The listing builds one solid part. Answer for the finished solid, in the listing's coordinates (mm). Face numbers are marked on the shaded views. A direction names the side the tool comes from. Round coordinates to 2 decimals unless told otherwise and drop trailing zeros. Write each loop counter-clockwise with the first axis right and the second up, starting at its lowest first coordinate (ties: lowest second). Pieces come first, ordered by that corner, then holes.
Item 1: Find the intervals of material crossed by probe 1 along X at (y, z) = (-1.6, 14); probe 2 along Y at (x, z) = (-30, -7.5); probe 3 along Z at (x, y) = (-9, -3), in increasing order.
Item 2: Each of these flat-tipped pins is pushed along its axis until it touches: pin 1 (2.5 mm diameter, centred on x = -51.5, y = -1.5, fed in from +Z); pin 2 (4 mm diameter, centred on x = -22.5, z = 0, fed in from +Y); pin 3 (4 mm diameter, centred on x = 0, z = 0, fed in from +Y); pin 4 (1.5 mm diameter, centred on x = 6, z = 37.5, fed in from -Y). Where does it stop, or does it pass through?
Item 3: Find section C-C on x = -51.75. Give the vertices of the cut face in (y, z).
Item 4: A tool of negligible diameter and unlimited length cuts with its end or side. For the marked faces 1 and 2, from which of +Z, -Z, +X, -X, +Y, -Y can it reach the whole face along a straight path? Write none if from no direction.
Item 5: Find section B-B on z = -14. Give the vertices of the cut face in (x, y), then the cut area to 3 significant figures.
Item 6: Find section D-D on x = 14. Give the vertices of the cut face in (y, z).
```python
from build123d import *

# Parameters (mm, degrees)
SKETCH1_R                               = 50
BOSS_EXTRUDE1_DEPTH                     = 4.5
BOSS_EXTRUDE2_DEPTH                     = 5
SKETCH4_R                               = 18
SKETCH4_R_2                             = 16
EXTRUDE_THIN1_DEPTH                     = 5
SKETCH7_R                               = 27
CUT_EXTRUDE1_DEPTH                      = 2
CBORE_FOR_M5_HEX_HEAD_BOLT2_D           = 5
CBORE_FOR_M5_HEX_HEAD_BOLT2_CBORE_D     = 13
CBORE_FOR_M5_HEX_HEAD_BOLT2_CBORE_DEPTH = 2
CUT_EXTRUDE2_DEPTH                      = 74.247866863
SKETCH11_R                              = 2.5
BOSS_EXTRUDE3_DEPTH                     = 4
SKETCH12_R                              = 1
CUT_EXTRUDE3_DEPTH                      = 74.764829018
EXTRUDE_THIN2_REACH                     = 75.765
SKETCH13_R                              = 2.5
SKETCH13_R_2                            = 1.5
CIRPATTERN1_COUNT                       = 4
SKETCH14_R                              = 1.25
CUT_EXTRUDE4_DEPTH                      = 74.247866863


with BuildPart() as part:
    # Sketch1 → Boss-Extrude1 (new body)
    with BuildSketch(Plane(origin=(0, 0, 0), x_dir=(1, 0, 0), z_dir=(0, 1, 0))):
        with Locations(Location((0, 0, 0), (0, 0, 270))):
            Circle(SKETCH1_R)
    extrude(amount=BOSS_EXTRUDE1_DEPTH)

    # Sketch3 → Boss-Extrude2 (add, symmetric)
    with BuildSketch(Plane.XY):
        with BuildLine():
            Line((0, 2.5), (-53, 2.5))
            Line((-53, 2.5), (-53, -2.25))
            ThreePointArc((-53, -2.25), (-51.75, -3.5), (-50.5, -2.25))
            Line((-50.5, -2.25), (-50.5, 0))
            Line((-50.5, 0), (0, 0))
            Line((0, 0), (0, 2.5))
        make_face()
    extrude(amount=BOSS_EXTRUDE2_DEPTH, both=True)

    # Sketch4 → Extrude-Thin1 (add)
    with BuildSketch(Plane.XZ):
        Circle(SKETCH4_R)
        Circle(SKETCH4_R_2, mode=Mode.SUBTRACT)
    extrude(amount=EXTRUDE_THIN1_DEPTH)

    # Sketch7 → Cut-Extrude1 (cut)
    with BuildSketch(Plane(origin=(0, 4.5, 0), x_dir=(1, 0, 0), z_dir=(0, 1, 0))):
        with Locations(Location((0, 0, 0), (0, 0, 270))):
            Circle(SKETCH7_R)
    extrude(amount=-CUT_EXTRUDE1_DEPTH, mode=Mode.SUBTRACT)

    # CBORE for M5 Hex Head Bolt2 (through all)
    with Locations(Plane(origin=(0, 2.5, 0), x_dir=(1, 0, 0), z_dir=(0, 1, 0))):
        with Locations((0, 0)):
            CounterBoreHole(CBORE_FOR_M5_HEX_HEAD_BOLT2_D / 2, CBORE_FOR_M5_HEX_HEAD_BOLT2_CBORE_D / 2, CBORE_FOR_M5_HEX_HEAD_BOLT2_CBORE_DEPTH)

    # Sketch10 → Cut-Extrude2 (cut, through all)
    with BuildSketch(Plane(origin=(0, 2.5, 0), x_dir=(1, 0, 0), z_dir=(0, 1, 0))):
        with BuildLine():
            Line((-21.405668752, 16.455921283), (-23.792893219, 19.550252532))
            ThreePointArc((-23.792893219, 19.550252532), (-28.035533906, 28.035533906), (-19.550252532, 23.792893219))
            Line((-19.550252532, 23.792893219), (-16.455921283, 21.405668752))
            ThreePointArc((-16.455921283, 21.405668752), (-19.091883092, 19.091883092), (-21.405668752, 16.455921283))
        make_face()
    cut_extrude2 = extrude(amount=CUT_EXTRUDE2_DEPTH, mode=Mode.SUBTRACT)

    # Sketch11 → Boss-Extrude3 (add)
    with BuildSketch(Plane(origin=(0, 2.5, 0), x_dir=(1, 0, 0), z_dir=(0, 1, 0))):
        with Locations(Location((-24.5, 24.5, 0), (0, 0, 270))):
            Circle(SKETCH11_R)
    boss_extrude3 = extrude(amount=BOSS_EXTRUDE3_DEPTH)

    # Sketch12 → Cut-Extrude3 (cut, through all)
    with BuildSketch(Plane(origin=(0, 6.5, 0), x_dir=(1, 0, 0), z_dir=(0, 1, 0))):
        with Locations(Location((-24.5, 24.5, 0), (0, 0, 270))):
            Circle(SKETCH12_R)
    cut_extrude3 = extrude(amount=-CUT_EXTRUDE3_DEPTH, mode=Mode.SUBTRACT)

    # Sketch13 → Extrude-Thin2 (add, up to next)
    with BuildSketch(Plane.XZ.offset(5), mode=Mode.PRIVATE) as extrude_thin2_sk1:
        with Locations((-14, 0)):
            Circle(SKETCH13_R)
        with Locations((-14, 0)):
            Circle(SKETCH13_R_2, mode=Mode.SUBTRACT)
    extrude_thin2_tool1 = extrude(extrude_thin2_sk1.sketch, amount=-EXTRUDE_THIN2_REACH, mode=Mode.PRIVATE) - part.part
    extrude_thin2 = extrude_thin2_tool1.solids().sort_by_distance((-16.429289, -5, 0))[0]
    add(extrude_thin2)

    # CirPattern1: Cut-Extrude2, Boss-Extrude3, Cut-Extrude3, Extrude-Thin2 ×4 about axis
    cirpattern1_axis = Axis((0, 0, 0), (0, 1, 0))
    add([cut_extrude2.rotate(cirpattern1_axis, i * 360 / CIRPATTERN1_COUNT) for i in range(1, CIRPATTERN1_COUNT)], mode=Mode.SUBTRACT)
    add([boss_extrude3.rotate(cirpattern1_axis, i * 360 / CIRPATTERN1_COUNT) for i in range(1, CIRPATTERN1_COUNT)])
    add([cut_extrude3.rotate(cirpattern1_axis, i * 360 / CIRPATTERN1_COUNT) for i in range(1, CIRPATTERN1_COUNT)], mode=Mode.SUBTRACT)
    add([extrude_thin2.rotate(cirpattern1_axis, i * 360 / CIRPATTERN1_COUNT) for i in range(1, CIRPATTERN1_COUNT)])

    # Sketch14 → Cut-Extrude4 (cut, through all)
    with BuildSketch(Plane(origin=(0, 2.5, 0), x_dir=(1, 0, 0), z_dir=(0, 1, 0))):
        with Locations(Location((-23, 0, 0), (0, 0, 270))):
            Circle(SKETCH14_R)
    extrude(amount=-CUT_EXTRUDE4_DEPTH, mode=Mode.SUBTRACT)


solid = part.part
```
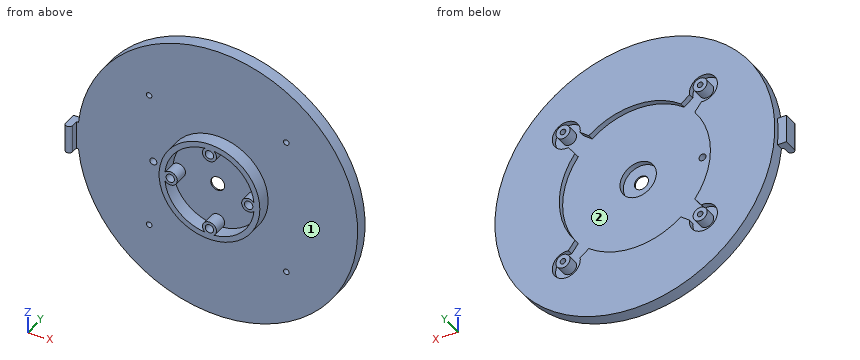
Check values:
1. probe 1: x = -11.31 to -7.75, -2.5 to -1.5, 1.5 to 2.5, 7.75 to 11.31
1. probe 2: y = 0 to 4.5
1. probe 3: z = -15.59 to -13.23, 13.23 to 15.59
2. pin 1: stops at z = 5
2. pin 2: stops at y = 2.5
2. pin 3: passes through
2. pin 4: stops at y = 0
3. outline: (-3.5, -5) - (2.5, -5) - (2.5, 5) - (-3.5, 5) - close
4. face 1: -Y
4. face 2: +Y
5. outline: (-48, 0) - (-11.31, 0) - (-11.31, -5) - (-7.75, -5) - (-7.75, 0) - (-2.5, 0) - (-2.5, -5) - (-1.5, -5) - (-1.5, 0) - (1.5, 0) - (1.5, -5) - (2.5, -5) - (2.5, 0) - (7.75, 0) - (7.75, -5) - (11.31, -5) - (11.31, 0) - (48, 0) - (48, 4.5) - (23.09, 4.5) - (23.09, 2.5) - (-23.09, 2.5) - (-23.09, 4.5) - (-48, 4.5) - close
5. area: 385 mm2
6. outline: (-5, -11.31) - (0, -11.31) - (0, -48) - (4.5, -48) - (4.5, -23.09) - (2.5, -23.09) - (2.5, 23.09) - (4.5, 23.09) - (4.5, 48) - (0, 48) - (0, 11.31) - (-5, 11.31) - (-5, 7.75) - (0, 7.75) - (0, 2.5) - (-5, 2.5) - (-5, 1.5) - (0, 1.5) - (0, -1.5) - (-5, -1.5) - (-5, -2.5) - (0, -2.5) - (0, -7.75) - (-5, -7.75) - close
